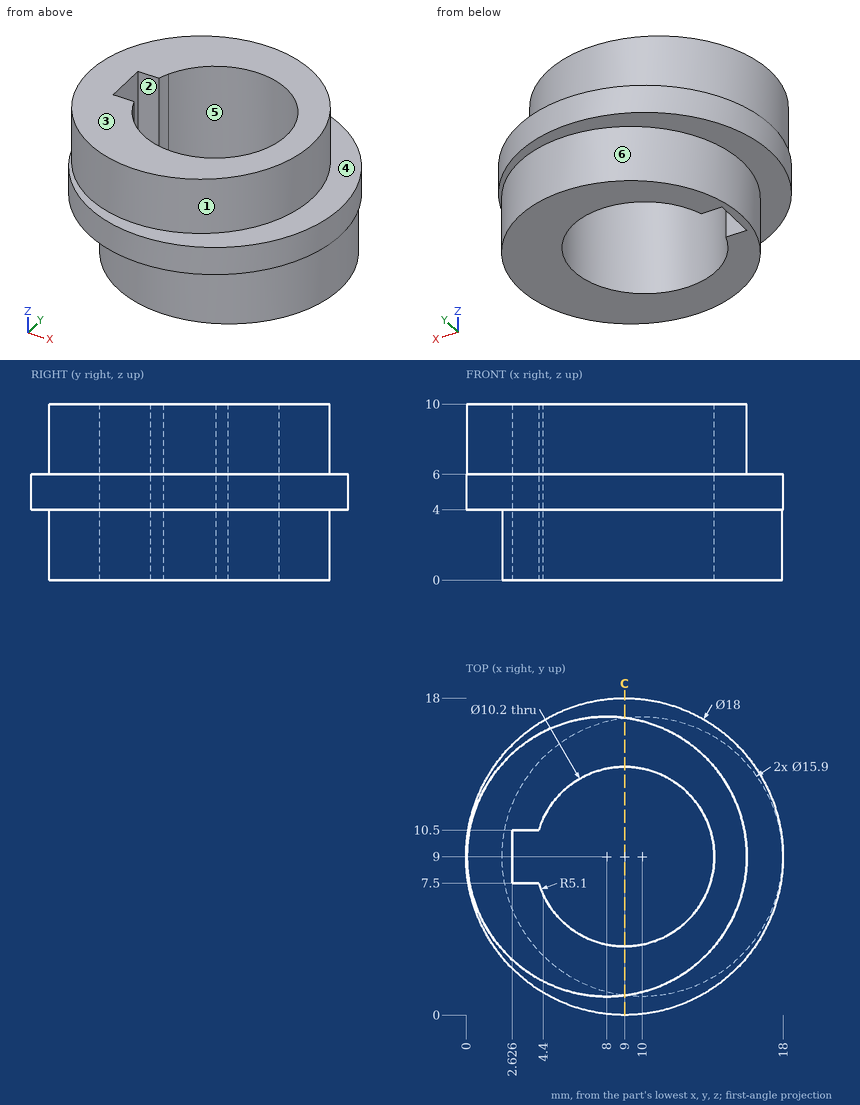
Study the drawing (mm; zero at the part's minimum x, y, z) and answer. A direction names the side the tool comes from. Give positions to 0.01 mm unless a question says otherwise; leave off trailing zeros. Order: outer loops, then holes, each group sorted by start corner. A loop starts at its lowest first (then second) coordinate and runs counter-clockwise, first axis right, second up. Notation, with made-up numbers: (-3.75, 69) - (48.25, 69) arc R14 ccw to (48.25, 87) - close; hole circle Ø4 at (60.25, -9). An arc over 180 degrees is marked (long way). Answer as CSV lines item,"result". Start each with the question number.
Q1. Given pin 1 Ø1.2 at (x, z) = (3.5, 5) entering from -Y; pin 2 Ø3 at (y, z) = (11.5, 6.5) entering from +X; pin 3 Ø1.5 at (y, z) = (9, 7.5) entering from +X; pin 4 Ø5 at (x, y) = (13.5, 16) entering from -Z, each flat-ended and moving along its own axis, determine where each tip first touches the part or whether it passes through.
Q2. Find the intervals of material crossed by L1, parallel to Y at x = 9, z = 5.25; L2, parallel to Z at x = 7.5, y = 1.25; L3, parallel to Z at x = 14.5, y = 2, in increasing order. Write a range as [from, to].
Q3. For the marked faces 1, 2 and 3, determine the directions among +Z, -Z, +X, -X, +Y, -Y from which every point of the face is accessible in a straight line to the end or side of a thin tool.
Q4. The mould has two halves that part along Y. Classify the marked faces 4, 5 and 6: +Y half, -Y half, draft (parallel to the pull), parting line (faces both ways), or undercut.
Q5. The part is cut by section C-C (x = 9). Write down the section's boundary in (y, z).
Check result:
1,pin 1,"stops at y = 1.45"
1,pin 2,"stops at x = 17.93"
1,pin 3,"stops at x = 15.95"
1,pin 4,"stops at z = 0"
2,L1,"y = [0, 3.9], [14.1, 18]"
2,L2,"z = [4, 10]"
2,L3,"z = [4, 6]"
3,face 1,"+Z"
3,face 2,"+Z, -Z"
3,face 3,"+Z, +X, -X, +Y, -Y"
4,face 4,"draft"
4,face 5,"undercut"
4,face 6,"parting line"
5,outline,"(0, 4) - (1.11, 4) - (1.11, 0) - (3.9, 0) - (3.9, 10) - (1.11, 10) - (1.11, 6) - (0, 6) - close; (14.1, 0) - (16.89, 0) - (16.89, 4) - (18, 4) - (18, 6) - (16.89, 6) - (16.89, 10) - (14.1, 10) - close"
